Job drawing, mm, ordinate dimensions from the low corner. One solid piece. A direction names the side the tool comes from. Round coordinates to 2 decimals unless told otherwise and drop trailing zeros. Loops run counter-clockwise (first coordinate to the right, second up) from the corner with the lowest first, then second, coordinate; pieces in that order, holes last.
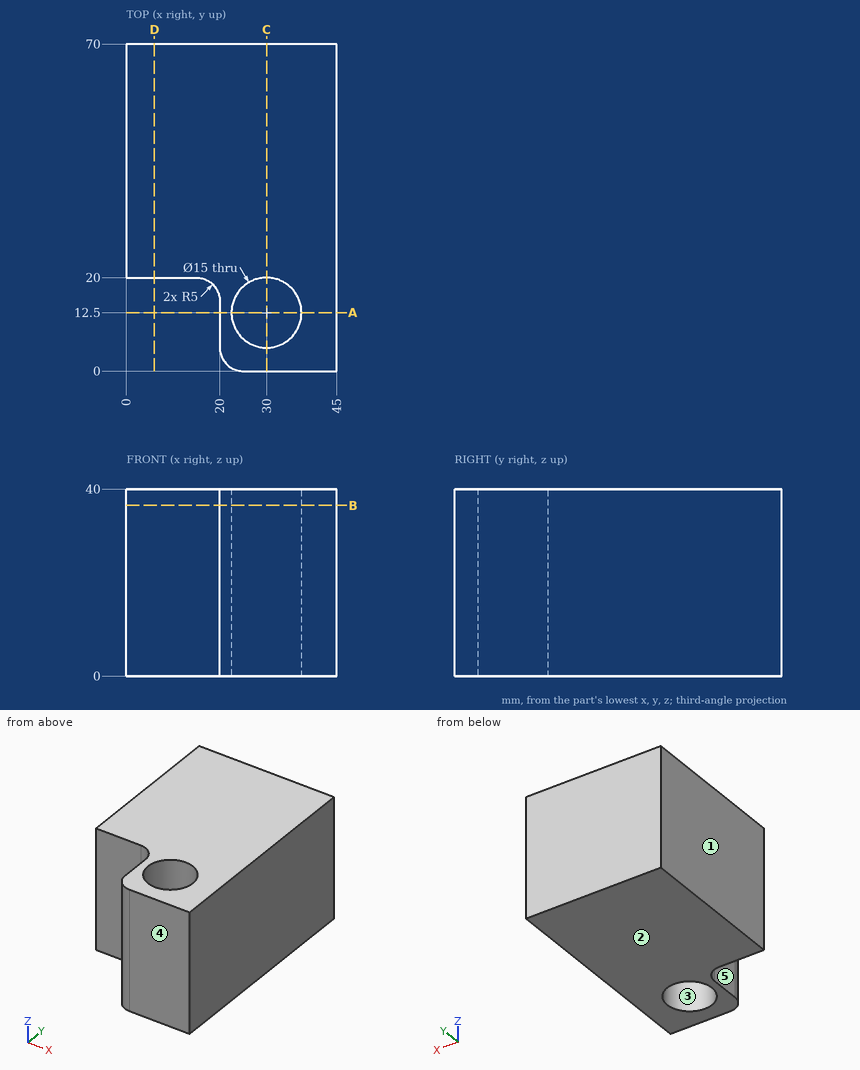
(1) Slice it at D-D on x = 6. List the corners of the cut face in (y, z).
Responses:
outline: (20, 0) - (70, 0) - (70, 40) - (20, 40) - close
(2) Pull direction X, two halves, no side cores. Call the marked faces 1, 2 and 3: +X half, -X half, draft (parallel to the pull), parting line (faces both ways), or undercut.
Responses:
face 1: -X half
face 2: draft
face 3: undercut
(3) Slice it at C-C on x = 30. List the corners of the cut face in (y, z), plus the area to 3 significant figures.
Responses:
outline: (0, 0) - (5, 0) - (5, 40) - (0, 40) - close; (20, 0) - (70, 0) - (70, 40) - (20, 40) - close
area: 2,200 mm2
(4) Which spindle directions (+Z, -Z, +X, -X, +Y, -Y) get a long thin tool onto all of the face, cutting with end or side? Do the marked faces 4 and 5. Say none if no direction does.
Responses:
face 4: +Z, -Z, +X, -X, -Y
face 5: +Z, -Z, -X, -Y
(5) Slice it at A-A on y = 12.5. List the corners of the cut face in (x, z), plus the area to 3 significant figures.
Responses:
outline: (20, 0) - (22.5, 0) - (22.5, 40) - (20, 40) - close; (37.5, 0) - (45, 0) - (45, 40) - (37.5, 40) - close
area: 400 mm2
(6) Probe line 1 (Y direction, x = 30, z = 15); line 2 (X direction, y = 12, z = 29); line 3 (Y direction, x = 32.5, z = 31). List the from-to ranges inside material, lowest first.
Responses:
line 1: y = 0 to 5, 20 to 70
line 2: x = 20 to 22.52, 37.48 to 45
line 3: y = 0 to 5.43, 19.57 to 70
(7) Slice it at B-B on z = 36.5. List the corners of the cut face in (x, y), plus the area to 3 significant figures.
Responses:
outline: (0, 20) - (15, 20) arc R5 cw to (20, 15) - (20, 5) arc R5 ccw to (25, 0) - (45, 0) - (45, 70) - (0, 70) - close; hole circle Ø15 at (30, 12.5)
area: 2,570 mm2
(8) Pin check, flat tips, straight feed: P1, Ø7.5, axis at x = 4.5, z = 24, coming from the -Y side; P2, Ø4, axis at x = 18.5, z = 33, coming from the -Y side; P3, Ø5, axis at y = 8.5, z = 28, coming from the -X side. Stop position of each tip, or through.
Responses:
P1: stops at y = 20
P2: stops at y = 2.82
P3: stops at x = 20
